The listing builds one solid part. Answer for the finished solid, in the listing's coordinates (mm). Face numbers are marked on the shaded views. Round coordinates to 2 decimals unless told otherwise and drop trailing zeros. Return JSON: item names as keys, results as strings. Group by question number.
(1) Find the intervals of material crossed by line 1 along X through (y, z) = (0, -105); line 2 along Z through (x, y) = (-214, -68.5); line 3 along Y through (x, z) = (-334.5, 116.5), in increasing order. Write a range as [from, to].
(2) Each of these flat-tipped pins is pushed along its axis until it touches: pin 1 (4 mm diameter, centred on x = -301.5, z = -45.5, fed in from +Y); pin 2 (2 mm diameter, centred on x = -284.5, z = -88, fed in from +Y); pin 3 (10 mm diameter, centred on x = -275, y = 8, fed in from +Z). Where does it stop, or does it pass through?
(3) Determine the mould class of the marked faces 1, 2 and 3 for opening direction Z: +Z half, -Z half, draft (parallel to the pull), parting line (faces both ways), or undercut.
```python
from build123d import *

# Parameters (mm, degrees)
F1_R   = 84.1375
F1_R_2 = 76.2


with BuildPart() as f2:
    # F2: sweep along a path in F0
    with BuildLine(Plane.XZ) as f2_path:
        Line((0, 168.275), (-92.539645279, 168.275))
        ThreePointArc((-92.539645279, 168.275), (-265.081021782, 96.806021782), (-336.55, -75.735354721))
        Line((-336.55, -75.735354721), (-336.55, -168.275))
    # F1 (on Right) → F2 (sweep)
    with BuildSketch(Plane.YZ):
        with Locations((0, 168.275)):
            Circle(F1_R)
        with Locations((0, 168.275)):
            Circle(F1_R_2, mode=Mode.SUBTRACT)
    sweep(path=f2_path.line)


solid = f2.part
```
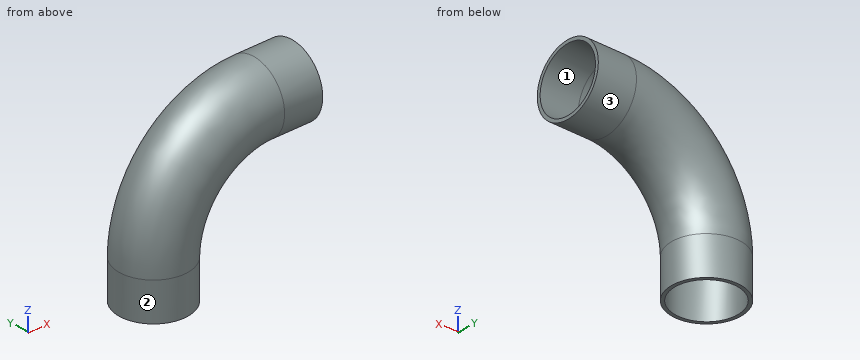
Working result:
{
 "1": {"line 1": "x = [-420.69, -412.75], [-260.35, -252.41]", "line 2": "z = [77.02, 96.35], [173.65, 190.76]", "line 3": "y = [-53.4, -39.74], [39.74, 53.4]"},
 "2": {"pin 1": "stops at y = 78.27", "pin 2": "stops at y = 66.88", "pin 3": "stops at z = 199.88"},
 "3": {"face 1": "undercut", "face 2": "draft", "face 3": "parting line"}
}
